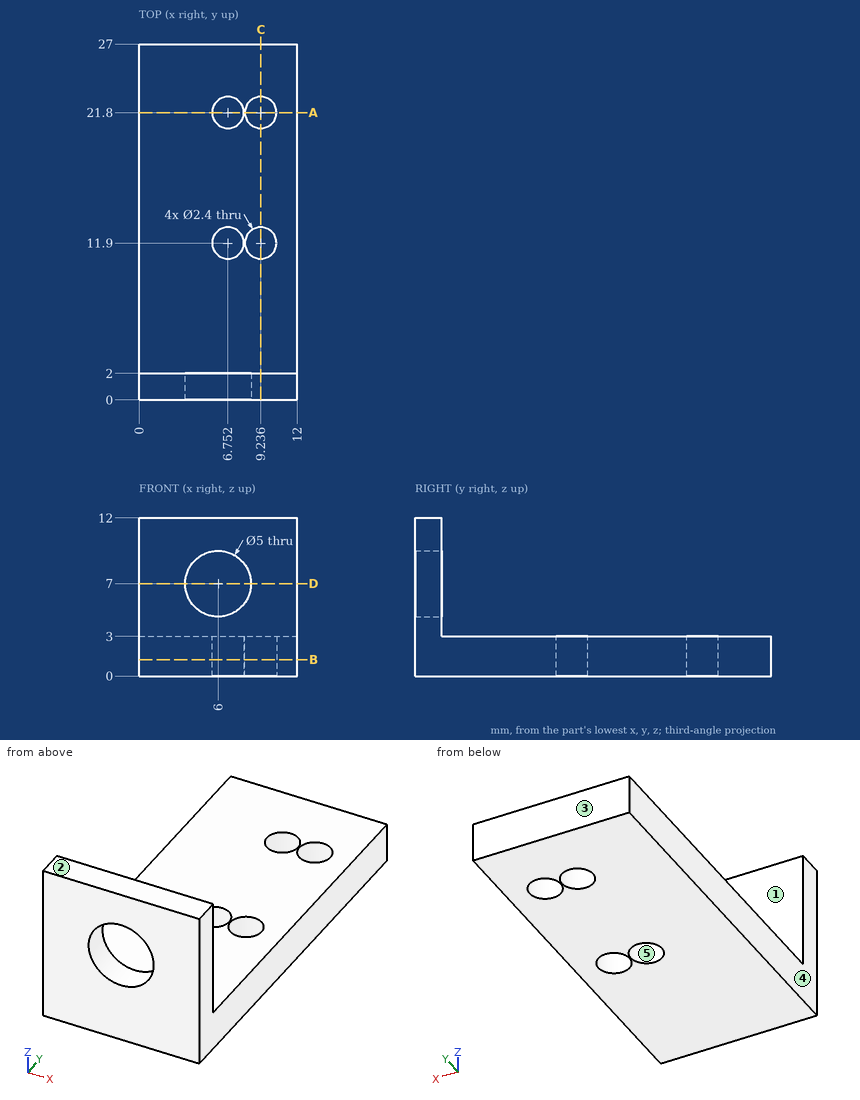
Geometry: see drawing. Coordinates: mm, zero at the bounding-box minimum. A direction names the side the tool comes from. Round coordinates to 2 decimals unless told otherwise and drop trailing zeros. Loops run counter-clockwise (first coordinate to the right, second up) from the corner with the lowest first, then second, coordinate; pieces in that order, holes last.
(1) Access query for the marked faces 1 and 2. Directions: +Z, -Z, +X, -X, +Y, -Y. A direction counts if a zero-diameter tool reaches every point of the face in a straight line with its end or side. Return the directions, or none.
From the geometry:
face 1: +Z, +X, -X, +Y
face 2: +Z, +X, -X, +Y, -Y
(2) Section query A-A (y = 21.8). Output: boundary loops of the cut face in (x, z), and give its area (3 significant figures).
From the geometry:
outline: (0, 0) - (5.55, 0) - (5.55, 3) - (0, 3) - close; (7.95, 0) - (8.04, 0) - (8.04, 3) - (7.95, 3) - close; (10.44, 0) - (12, 0) - (12, 3) - (10.44, 3) - close
area: 21.6 mm2
(3) Section query B-B (z = 1.25). Output: boundary loops of the cut face in (x, y).
From the geometry:
outline: (0, 0) - (12, 0) - (12, 27) - (0, 27) - close; hole circle Ø2.4 at (6.75, 11.9); hole circle Ø2.4 at (6.75, 21.8); hole circle Ø2.4 at (9.24, 11.9); hole circle Ø2.4 at (9.24, 21.8)
(4) Section query C-C (x = 9.25). Output: boundary loops of the cut face in (y, z), and give its area (3 significant figures).
From the geometry:
outline: (0, 0) - (10.7, 0) - (10.7, 3) - (2, 3) - (2, 12) - (0, 12) - close; (13.1, 0) - (20.6, 0) - (20.6, 3) - (13.1, 3) - close; (23, 0) - (27, 0) - (27, 3) - (23, 3) - close
area: 84.6 mm2
(5) Section query D-D (z = 7). Output: boundary loops of the cut face in (x, y).
From the geometry:
outline: (0, 0) - (3.5, 0) - (3.5, 2) - (0, 2) - close; (8.5, 0) - (12, 0) - (12, 2) - (8.5, 2) - close
(6) Pull-direction query (X, two-part tool) for the marked faces 3, 4 and 5; classes: +X half, -X half, draft (parallel to the pull), parting line (faces both ways), or undercut.
From the geometry:
face 3: draft
face 4: -X half
face 5: undercut
(7) Material intervals for probe 1 along X at (y, z) = (0.6, 7); probe 2 along Z at (x, y) = (6, 0.5); probe 3 along Y at (x, z) = (2.5, 3.5), sorted ascending.
From the geometry:
probe 1: x = 0 to 3.5, 8.5 to 12
probe 2: z = 0 to 4.5, 9.5 to 12
probe 3: y = 0 to 2
(8) Contact query for flat-ended pins moving along their axis: pin 1 Ø3 at (x, y) = (9.24, 11.9) entering from +Z; pin 2 Ø2 at (x, z) = (9, 9.5) entering from +Y. Output: stop coordinate, or through.
From the geometry:
pin 1: stops at z = 3
pin 2: stops at y = 2
